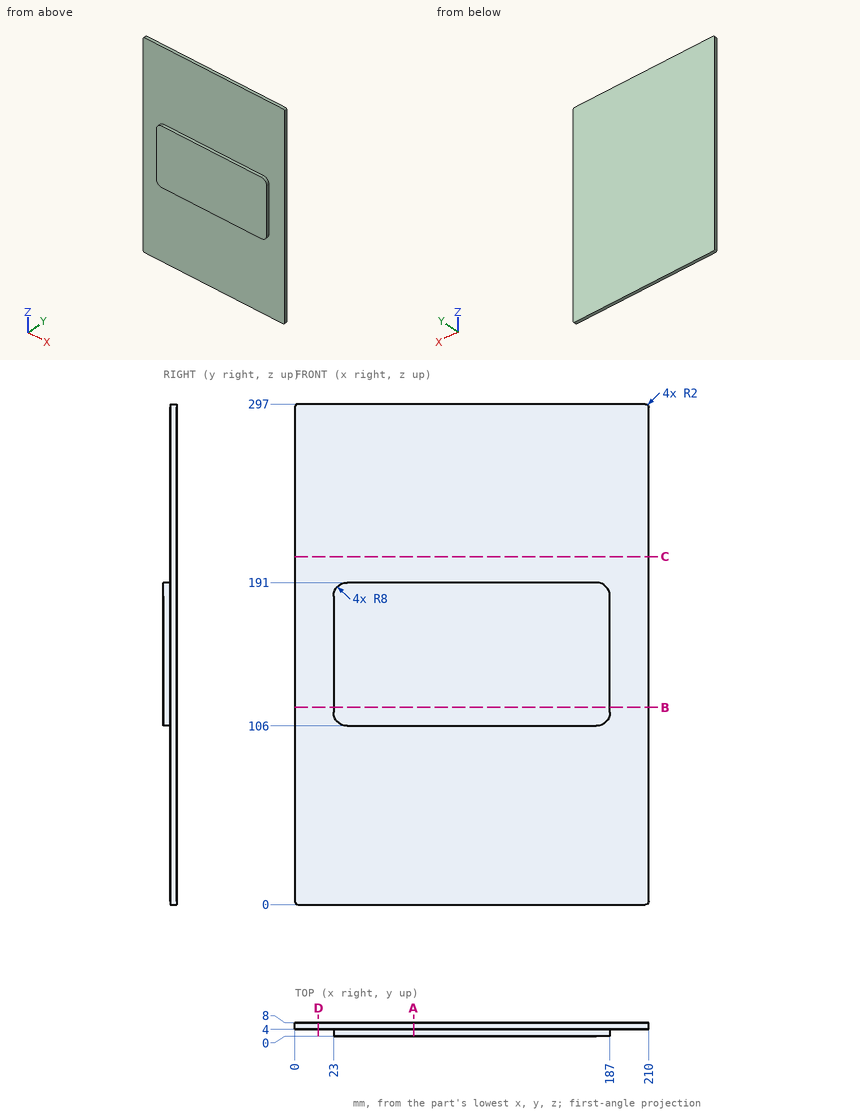
Source: three-view drawing plus pictorial views. Frame: mm from the lowest corner of the part. Give positions to 0.01 mm unless a question says otherwise; leave off trailing zeros. Loops run counter-clockwise (first coordinate to the right, second up) from the corner with the lowest first, then second, coordinate; pieces in that order, holes last. Notation, with made-up numbers: M -0.5,77.25 L 52.5,77.25 A30 cw 52.5,111.25 Z; hole C -10.75,72.25 d4. An arc over 180 degrees is marked long. Put each result on its own line as item: value.
Q1. Section D-D (x = 14). Return the cut outline in (y, z).
Response values:
outline: M 4,0 L 8,0 L 8,297 L 4,297 Z
Q2. Section B-B (z = 117). Return the cut outline in (x, y), and give its area (3 significant figures).
Response values:
outline: M 0,4 L 23,4 L 23,0 L 187,0 L 187,4 L 210,4 L 210,8 L 0,8 Z
area: 1,500 mm²
Q3. Section A-A (x = 70.5). Return the cut outline in (y, z), and give its area (3 significant figures).
Response values:
outline: M 0,106 L 4,106 L 4,0 L 8,0 L 8,297 L 4,297 L 4,191 L 0,191 Z
area: 1,530 mm²
Q4. Pin query (flat end, axial travel): P1, Ø1.5, axis at x = 131, y = 2, coming from the +Z side; P2, Ø1.2, axis at x = 116.5, y = 2, coming from the -Z side; P3, Ø3, axis at x = 92.5, z = 159, coming from the -Y side; P4, Ø4, axis at x = 101.5, z = 87.5, coming from the -Y side. Return the tip coordinate at first contact, or that it passes through.
Response values:
P1: stops at z = 191
P2: stops at z = 106
P3: stops at y = 0
P4: stops at y = 4
Q5. Section C-C (z = 206.5). Return the cut outline in (x, y).
Response values:
outline: M 0,4 L 210,4 L 210,8 L 0,8 Z
Q6. Line query: probe 1 along Y at (x, z) = (176, 58.5); probe 2 along X at (y, z) = (1.25, 126); probe 3 along Z at (x, y) = (31.5, 3). Output: solid intervals per line, ascending. Write a range as [from, to].
Response values:
probe 1: y = [4, 8]
probe 2: x = [23, 187]
probe 3: z = [106, 191]
